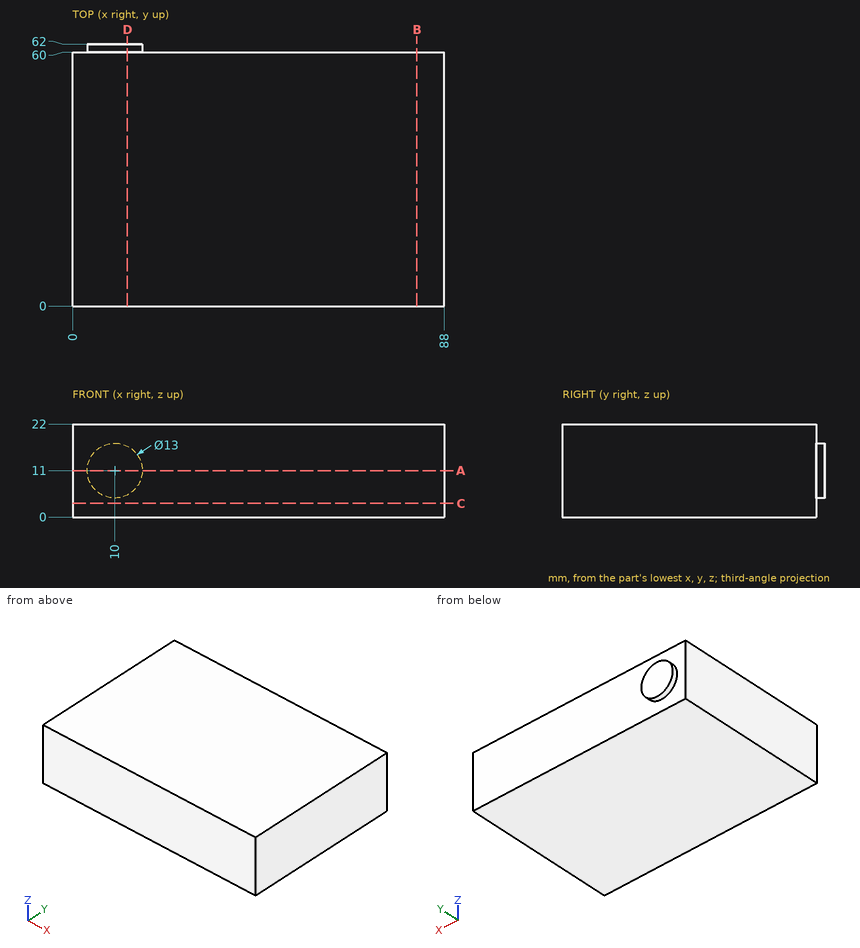
Job drawing, mm, ordinate dimensions from the low corner. One solid piece. Coordinates: 2 decimals unless noted, no trailing zeros. Order: outer loops, then holes, each group sorted by start corner. A loop starts at its lowest first (then second) coordinate and runs counter-clockwise, first axis right, second up. Notation, with made-up numbers: M 46,46 L 97,46 A23 ccw 97,59 Z; hole C -5,26.25 d7. An arc over 180 degrees is marked long. One line per question, with ' | ' between items.
Q1. Pin check, flat tip, straight feed: P1, Ø1.5, axis at x = 61, z = 18, coming from the +Y side. Stop position of the tip, or through.
A:
P1: stops at y = 60
Q2. Slice it at A-A (z = 11). Give the cut face in (x, y), and give its area (3 significant figures).
A:
outline: M 0,0 L 88,0 L 88,60 L 16.5,60 L 16.5,62 L 3.5,62 L 3.5,60 L 0,60 Z | area: 5,310 mm^2
Q3. Slice it at C-C (z = 3.25). Give the cut face in (x, y), and give its area (3 significant figures).
A:
outline: M 0,0 L 88,0 L 88,60 L 0,60 Z | area: 5,280 mm^2
Q4. Drill centre line: line 1 (Y direction, x = 37, z = 19.5). Where is it in solid material? Low to high.
A:
line 1: y = 0 to 60
Q5. Slice it at B-B (x = 81.5). Give the cut face in (y, z).
A:
outline: M 0,0 L 60,0 L 60,22 L 0,22 Z
Q6. Slice it at D-D (x = 13). Give the cut face in (y, z), and give its area (3 significant figures).
A:
outline: M 0,0 L 60,0 L 60,5.23 L 62,5.23 L 62,16.77 L 60,16.77 L 60,22 L 0,22 Z | area: 1,340 mm^2
